Geometry check sheet. Reference: the model listing, model coordinates, mm. Face numbers are marked on the shaded views. A direction names the side the tool comes from. Coordinates: 2 decimals unless noted, no trailing zeros. Loops run counter-clockwise (first coordinate to the right, second up) from the corner with the lowest first, then second, coordinate; pieces in that order, holes last.
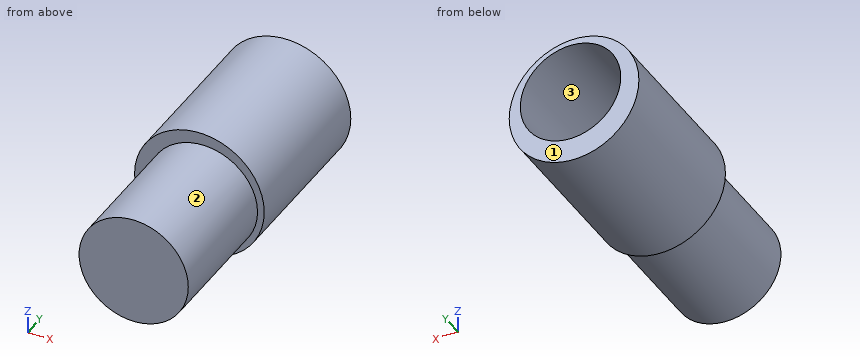
from build123d import *

# Parameters (mm, degrees)
F0_R     = 50.0856425189
F1_DEPTH = 101.6
F2_R     = 42.1792579473
F3_DEPTH = 101.6
F4_DEPTH = 25.4
F5_R     = 38.8092501819
F6_DEPTH = 101.6


with BuildPart() as f1:
    # F0 (on Front) → F1 (new body)
    with BuildSketch(Plane.XZ):
        with Locations((-2.7341553941, 9.0658813715)):
            Circle(F0_R)
    extrude(amount=F1_DEPTH)

    # F2 (on face) → F3 (join)
    with BuildSketch(Plane.XZ.offset(101.6)):
        with Locations((0, 7.6268524863)):
            Circle(F2_R)
    extrude(amount=F3_DEPTH)

    # F4 (add): a face of the model
    f4_faces = [f1.faces().sort_by_distance(p)[0] for p in [
        (-2.7341553941, 0, 9.0658813715),
    ]]
    extrude(f4_faces, amount=F4_DEPTH)

    # F5 (on face) → F6 (cut)
    with BuildSketch(Plane(origin=(0, 25.4, 0), x_dir=(-1, 0, 0), z_dir=(0, 1, 0))):
        with Locations((0, 15.973219648)):
            Circle(F5_R)
    extrude(amount=-F6_DEPTH, mode=Mode.SUBTRACT)


solid = f1.part
1) Section check C-C on y = 6.5. Record the cut outline in (x, z), and give its area (3 significant figures).
Data:
outline: circle Ø100.17 at (-2.73, 9.07); hole circle Ø77.62 at (0, 15.97)
area: 3,150 mm2
2) Section check A-A on x = 32. Record the cut outline in (y, z), and give its area (3 significant figures).
Data:
outline: (-203.2, -19.85) - (-101.6, -19.85) - (-101.6, -27.02) - (25.4, -27.02) - (25.4, -5.98) - (-76.2, -5.98) - (-76.2, 37.93) - (25.4, 37.93) - (25.4, 45.15) - (-101.6, 45.15) - (-101.6, 35.11) - (-203.2, 35.11) - close
area: 10,300 mm2
3) Access from +Z, -Z, +X, -X, +Y, -Y to the whole of each face (thin tool, end or side, straight path). Record for the marked faces 1, 2 and 3.
Data:
face 1: +Z, -Z, +X, -X, +Y
face 2: -Y
face 3: +Y
4) Section check B-B on z = 22.5. Record the cut outline in (x, y).
Data:
outline: (-50.98, -101.6) - (-39.47, -101.6) - (-39.47, -203.2) - (39.47, -203.2) - (39.47, -101.6) - (45.52, -101.6) - (45.52, 25.4) - (38.26, 25.4) - (38.26, -76.2) - (-38.26, -76.2) - (-38.26, 25.4) - (-50.98, 25.4) - close
5) Material ranges on probe 1 along Z at (x, y) = (0, 3); probe 2 along Y at (x, z) = (-2.5, 26); probe 3 along X at (y, z) = (-54.5, -20), recorded low to high.
Data:
probe 1: z = -40.95 to -22.84, 54.78 to 59.08
probe 2: y = -203.2 to -76.2
probe 3: x = -43.52 to -14.56, 14.56 to 38.05
6) Depth check by flat-ended pin: pin 1 (4 mm diameter, centred on y = -1.5, z = -13, fed in from -X); pin 2 (12 mm diameter, centred on x = -13.5, y = -140.5, fed in from -Z); pin 3 (12 mm diameter, centred on x = -1.5, y = -111.5, fed in from +Z). Enter the tip coordinate at first touch or a pass-through.
Data:
pin 1: stops at x = -48.62
pin 2: stops at z = -33.88
pin 3: stops at z = 49.81
7) Section check D-D on y = -95. Record the cut outline in (x, z), and give its area (3 significant figures).
Data:
outline: circle Ø100.17 at (-2.73, 9.07)
area: 7,880 mm2
